Part model, mm, in its own coordinate system. A direction names the side the tool comes from. Coordinates: 2 decimals unless noted, no trailing zeros. Loops run counter-clockwise (first coordinate to the right, second up) from the corner with the lowest first, then second, coordinate; pieces in that order, holes last. Notation, with made-up numbers: M -6,56.5 L 41,56.5 A23 ccw 41,69.5 Z; hole C 68.25,-3 d5. An arc over 180 degrees is marked long. Answer as a JSON object with one key per item and string values. Group by question number.
1. 3-axis set-ups, long thin cutter, end or side, ignore diameter. For faces 1 (the face through (44.5, 54, -104)), 2 (the face through (1, 92.696, -98)), 3 (the face through (-30.23, 20.6, -19.47)), 4 (the face through (5, 93, -74.633)): which of +Z, -Z, +X, -X, +Y, -Y reach the whole face in a straight line?
2. Saw through at D-D on z = -104. Write the cut outline in (x, y).
3. Saw through at B-B on z = -25. Write the cut outline in (x, y).
4. Mould opens along Z. For faces 5 (the face through (47.95, 46.53, -64.68)), 6 (the face through (33.09, 20.6, -30.53)), 7 (the face through (-41.5, 54, -106)) say: released by +Z, released by -Z, zero draft, split by the parting line, or undercut.
5. Drop flat-ended pins along their axis: pin 1 Ø12 at (x, z) = (-11.5, -94) entering from -Y; pin 2 Ø4 at (x, y) = (16.5, 14) entering from -Z. Give the stop position or say it passes through.
6. Saw through at C-C on x = 1.5. Write the cut outline in (y, z), then the cut area to 3 significant figures.
7. Saw through at A-A on y = 58. Write the cut outline in (x, z).
8. Drill centre lines: L1, parallel to X at y = 61, z = -130; L2, parallel to X at y = 2, z = -31; L3, parallel to Z at x = 1.5, y = 94.5. Where is each one in solid material? Low to high.
from build123d import *

# Parameters (mm, degrees)
SKETCH1_W            = 100
SKETCH1_H            = 50
BOSS_EXTRUDE1_DEPTH  = 5
SKETCH2_W            = 7
SKETCH2_H            = 50
BOSS_EXTRUDE2_DEPTH  = 55
BOSS_EXTRUDE3_DEPTH  = 7
BOSS_EXTRUDE8_DEPTH  = 7
SKETCH14_W           = 80.726202609
SKETCH14_H           = 40
BOSS_EXTRUDE11_DEPTH = 7
SKETCH15_W           = 80.726202609
SKETCH15_H           = 40
BOSS_EXTRUDE12_DEPTH = 7
SKETCH24_W           = 100
SKETCH24_H           = 80.726202609
BOSS_EXTRUDE21_DEPTH = 5
SKETCH25_R           = 7
CUT_EXTRUDE5_DEPTH   = 101
SKETCH26_R           = 15
CUT_EXTRUDE6_DEPTH   = 5
BOSS_EXTRUDE22_REACH = 102
SKETCH30_R           = 2.25
SKETCH32_R           = 7.5
BOSS_EXTRUDE23_DEPTH = 23
SKETCH33_R           = 7.5
BOSS_EXTRUDE24_DEPTH = 23


with BuildPart() as part:
    # Sketch1 → Boss-Extrude1 (new body)
    with BuildSketch(Plane.XY):
        with Locations((1.428571429, 15.535714286)):
            Rectangle(SKETCH1_W, SKETCH1_H)
    extrude(amount=BOSS_EXTRUDE1_DEPTH)

    # Sketch2 → Boss-Extrude2 (add)
    with BuildSketch(Plane.XY):
        with Locations((47.928571429, 15.535714286)):
            Rectangle(SKETCH2_W, SKETCH2_H)
        with Locations((-45.071428571, 15.535714286)):
            Rectangle(SKETCH2_W, SKETCH2_H)
    extrude(amount=-BOSS_EXTRUDE2_DEPTH)

    # Sketch3 → Boss-Extrude3 (add)
    with BuildSketch(Plane(origin=(44.5, 0, 0), x_dir=(0, 0, -1), z_dir=(1, 0, 0))):
        Polygon((55, 40.535714286), (74.633488262, 52.696256729), (155.359690871, 52.696256729), (55, -9.464285714), align=None)
    extrude(amount=BOSS_EXTRUDE3_DEPTH)

    # Sketch11 → Boss-Extrude8 (add)
    with BuildSketch(Plane.ZY.offset(41.5)):
        Polygon((-55, -9.464285714), (-55, 40.535714286), (-74.633488262, 52.696256729), (-155.359690871, 52.696256729), align=None)
    extrude(amount=BOSS_EXTRUDE8_DEPTH)

    # Sketch14 → Boss-Extrude11 (add)
    with BuildSketch(Plane.ZY.offset(41.5)):
        with Locations((-114.996589567, 72.696256729)):
            Rectangle(SKETCH14_W, SKETCH14_H)
    extrude(amount=BOSS_EXTRUDE11_DEPTH)

    # Sketch15 → Boss-Extrude12 (add)
    with BuildSketch(Plane(origin=(44.5, 0, 0), x_dir=(0, 0, -1), z_dir=(1, 0, 0))):
        with Locations((114.996589567, 72.696256729)):
            Rectangle(SKETCH15_W, SKETCH15_H)
    extrude(amount=BOSS_EXTRUDE12_DEPTH)

    # Sketch24 → Boss-Extrude21 (add)
    with BuildSketch(Plane(origin=(0, 92.696256729, 0), x_dir=(1, 0, 0), z_dir=(0, 1, 0))):
        with Locations((1.5, 114.996589567)):
            Rectangle(SKETCH24_W, SKETCH24_H)
    extrude(amount=BOSS_EXTRUDE21_DEPTH)

    # Sketch25 → Cut-Extrude5 (cut, through all)
    with BuildSketch(Plane.ZY.offset(48.5)):
        with Locations((-114.996589567, 75.196256729)):
            Circle(SKETCH25_R)
    extrude(amount=-CUT_EXTRUDE5_DEPTH, mode=Mode.SUBTRACT)

    # Sketch26 → Cut-Extrude6 (cut)
    with BuildSketch(Plane.XZ.offset(-92.696256729)):
        with Locations((1.5, -114.996589567)):
            Circle(SKETCH26_R)
    extrude(amount=-CUT_EXTRUDE6_DEPTH, mode=Mode.SUBTRACT)

    # Sketch30 → Boss-Extrude22 (add, up to next)
    with BuildSketch(Plane(origin=(51.428571429, 0, 0), x_dir=(0, 0, -1), z_dir=(1, 0, 0)), mode=Mode.PRIVATE) as boss_extrude22_sk1:
        with Locations((25, 15.535714286)):
            Circle(SKETCH30_R)
    boss_extrude22_tool1 = extrude(boss_extrude22_sk1.sketch, amount=-BOSS_EXTRUDE22_REACH, mode=Mode.PRIVATE) - part.part
    add(boss_extrude22_tool1.solids().sort_by_distance((51.428571, 15.535714, -25))[0])

    # Sketch32 → Boss-Extrude23 (add)
    with BuildSketch(Plane.ZY.offset(-44.428571429)):
        with Locations((-25, 15.535714286)):
            Circle(SKETCH32_R)
    extrude(amount=BOSS_EXTRUDE23_DEPTH)

    # Sketch33 → Boss-Extrude24 (add)
    with BuildSketch(Plane(origin=(-41.571428571, 0, 0), x_dir=(0, 0, -1), z_dir=(1, 0, 0))):
        with Locations((25, 15.535714286)):
            Circle(SKETCH33_R)
    extrude(amount=BOSS_EXTRUDE24_DEPTH)


solid = part.part
Outcome:
{
 "1": {"face 1": "-Z, -Y", "face 2": "+Z, -Z, -Y", "face 3": "none", "face 4": "+Z, +X, -X, +Y"},
 "2": {"outline": "M -48.5,20.89 L -41.5,20.89 L -41.5,92.7 L -8.7,92.7 L -8.7,97.7 L -48.5,97.7 Z; M 11.7,92.7 L 44.5,92.7 L 44.5,20.89 L 51.5,20.89 L 51.5,97.7 L 11.7,97.7 Z"},
 "3": {"outline": "M -48.57,-9.46 L -41.57,-9.46 L -41.57,8.04 L -18.57,8.04 L -18.57,13.29 L 21.43,13.29 L 21.43,8.04 L 44.43,8.04 L 44.43,-9.46 L 51.43,-9.46 L 51.43,40.54 L 44.43,40.54 L 44.43,23.04 L 21.43,23.04 L 21.43,17.79 L -18.57,17.79 L -18.57,23.04 L -41.57,23.04 L -41.57,40.54 L -48.57,40.54 Z"},
 "4": {"face 5": "released by +Z", "face 6": "undercut", "face 7": "zero draft"},
 "5": {"pin 1": "stops at y = 92.7", "pin 2": "stops at z = -27.25"},
 "6": {"outline": "M -9.46,0 L 40.54,0 L 40.54,5 L -9.46,5 Z; C 15.54,-25 d4.5; M 92.7,-155.36 L 97.7,-155.36 L 97.7,-130 L 92.7,-130 Z; M 92.7,-100 L 97.7,-100 L 97.7,-74.63 L 92.7,-74.63 Z", "area": "520 mm²"},
 "7": {"outline": "M -48.5,-155.36 L -41.5,-155.36 L -41.5,-74.63 L -48.5,-74.63 Z; M 44.5,-155.36 L 51.5,-155.36 L 51.5,-74.63 L 44.5,-74.63 Z"},
 "8": {"L1": "x = -48.5 to -41.5, 44.5 to 51.5", "L2": "x = -48.57 to -41.57, 44.43 to 51.43", "L3": "z = -155.36 to -130, -100 to -74.63"}
}
